Build history of the part. All positions in model axes, mm. Face numbers are marked on the shaded views. A direction names the side the tool comes from. Round coordinates to 2 decimals unless told otherwise and drop trailing zeros. Write each loop counter-clockwise with the first axis right and the second up, starting at its lowest first coordinate (ties: lowest second). Pieces come first, ordered by that corner, then holes. Notation, with made-up numbers: M 5,54.5 L 25,54.5 A26 ccw 25,78.5 Z; hole C 3,-36.75 d3. An arc over 180 degrees is marked long. Use a Markdown table: item, result.
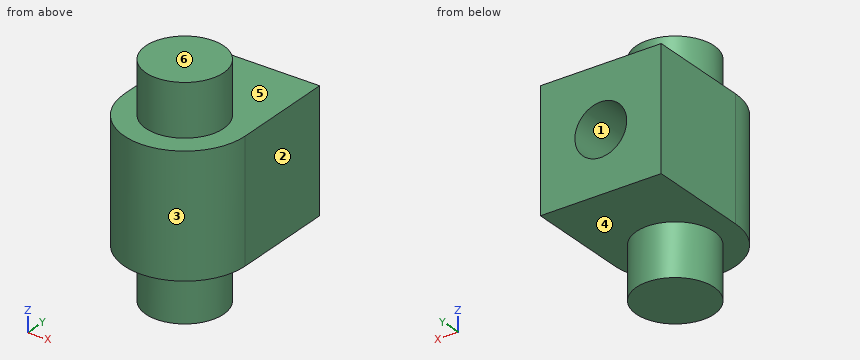
from build123d import *

# Parameters (mm, degrees)
EXTRUDE_1_DEPTH     = 7
SKETCH_3_R          = 2.25
EXTRUDE_2_DEPTH     = 3
EXTRUDE_START       = 3
SKETCH_4_R          = 2.25
EXTRUDE_3_DEPTH     = 3
SKETCH_5_R          = 1.5
CUT_EXTRUDE_4_DEPTH = 5


with BuildPart() as part:
    # 草圖1 → 伸長1 (new body)
    with BuildSketch(Plane.XY):
        with BuildLine():
            Line((-3.5, 0), (-3.5, 6))
            Line((-3.5, 6), (3.5, 6))
            Line((3.5, 6), (3.5, 0))
            ThreePointArc((3.5, 0), (0, -3.5), (-3.5, 0))
        make_face()
    extrude(amount=EXTRUDE_1_DEPTH)

    # 草圖3 → 伸長2 (add)
    with BuildSketch(Plane.XY.offset(7)):
        Circle(SKETCH_3_R)
    extrude(amount=EXTRUDE_2_DEPTH)

    # 草圖4 → 伸長3 (add)
    with BuildSketch(Plane(origin=(0, 0, 0), x_dir=(-1, 0, 0), z_dir=(0, 0, -1)).offset(EXTRUDE_START)):
        with Locations(Location((0, 0, 0), (0, 0, 180))):
            Circle(SKETCH_4_R)
    extrude(amount=-EXTRUDE_3_DEPTH)

    # 草圖5 → 伸長4 (cut)
    with BuildSketch(Plane(origin=(0, 6, 0), x_dir=(1, 0, 0), z_dir=(0, 1, 0))):
        with Locations(Location((0, -3.5, 0), (0, 0, 270))):
            Circle(SKETCH_5_R)
    extrude(amount=-CUT_EXTRUDE_4_DEPTH, mode=Mode.SUBTRACT)


solid = part.part
Q1. Drop flat-ended pins along their axis: P1, Ø1, axis at x = 0.5, y = 3, coming from the +Z side; P2, Ø0.9, axis at x = 0, z = 3, coming from the +Y side. Give the stop position or say it passes through.
Response values:
| item | result |
|---|---|
| P1 | stops at z = 7 |
| P2 | stops at y = 1 |
Q2. Cut at A-A on y = 4.75. Give the cut face in (x, z).
Response values:
| item | result |
|---|---|
| outline | M -3.5,0 L 3.5,0 L 3.5,7 L -3.5,7 Z; hole C 0,3.5 d3 |
Q3. Cut at B-B on z = 3.5. Give the cut face in (x, y).
Response values:
| item | result |
|---|---|
| outline | M -3.5,0 A3.5 ccw 3.5,0 L 3.5,6 L 1.5,6 L 1.5,1 L -1.5,1 L -1.5,6 L -3.5,6 Z |
Q4. Cut at C-C on x = -0.5. Give the cut face in (y, z).
Response values:
| item | result |
|---|---|
| outline | M -3.46,0 L -2.19,0 L -2.19,-3 L 2.19,-3 L 2.19,0 L 6,0 L 6,2.09 L 1,2.09 L 1,4.91 L 6,4.91 L 6,7 L 2.19,7 L 2.19,10 L -2.19,10 L -2.19,7 L -3.46,7 Z |
Q5. Two-plate mould, pull along X, no slides. Class the marked faces 1, 2 and 3: +X half, -X half, draft (parallel to the pull), parting line (faces both ways), or undercut.
Response values:
| item | result |
|---|---|
| face 1 | undercut |
| face 2 | +X half |
| face 3 | parting line |
Q6. Drill centre lines: L1, parallel to X at y = 3.75, z = 3.5; L2, parallel to Z at x = -2.25, y = -1.5; L3, parallel to Z at x = -0.5, y = 5.25. Where is each one in solid material? Low to high.
Response values:
| item | result |
|---|---|
| L1 | x = -3.5 to -1.5, 1.5 to 3.5 |
| L2 | z = 0 to 7 |
| L3 | z = 0 to 2.09, 4.91 to 7 |
Q7. Cut at D-D on y = 0.75. Give the cut face in (x, z), and give its area (3 significant figures).
Response values:
| item | result |
|---|---|
| outline | M -3.5,0 L -2.12,0 L -2.12,-3 L 2.12,-3 L 2.12,0 L 3.5,0 L 3.5,7 L 2.12,7 L 2.12,10 L -2.12,10 L -2.12,7 L -3.5,7 Z |
| area | 74.5 mm2 |
Q8. Which spindle directions (+Z, -Z, +X, -X, +Y, -Y) get a long thin tool onto all of the face, cutting with end or side? Do the marked faces 4, 5 and 6. Say none if no direction does.
Response values:
| item | result |
|---|---|
| face 4 | -Z |
| face 5 | +Z |
| face 6 | +Z, +X, -X, +Y, -Y |
